Check sheet for the modelled part. Datum: model origin and axes. Units: mm. A direction names the side the tool comes from. Coordinates: 2 decimals unless noted, no trailing zeros. Loops run counter-clockwise (first coordinate to the right, second up) from the corner with the lowest first, then second, coordinate; pieces in that order, holes last. Notation, with made-up numbers: (-17, 11.25) -> (24, 11.25) arc R30 ccw to (24, 33.25) -> close; hole circle Ø10 at (34, -20.75). An arc over 180 degrees is marked (long way). Use one line per item in the form item = value.
from build123d import *

# Parameters (mm, degrees)
SKETCH2_W           = 127
SKETCH2_H           = 177.8
BOSS_EXTRUDE2_DEPTH = 5.08
SKETCH3_W           = 5.08
SKETCH3_H           = 25.4
CUT_EXTRUDE1_DEPTH  = 5.08
LPATTERN1_COUNT     = 5
LPATTERN1_PITCH     = 43.18
SKETCH4_W           = 5.08
SKETCH4_H           = 25.4
CUT_EXTRUDE2_DEPTH  = 5.08
LPATTERN2_COUNT     = 4
LPATTERN2_PITCH     = 43.18
SKETCH5_W           = 25.4
SKETCH5_H           = 5.08
CUT_EXTRUDE3_DEPTH  = 5.08
LPATTERN3_COUNT     = 3
LPATTERN3_PITCH     = 38.1
SKETCH6_W           = 25.4
SKETCH6_H           = 5.08
CUT_EXTRUDE4_DEPTH  = 5.08
LPATTERN4_COUNT     = 3
LPATTERN4_PITCH     = 38.1
SKETCH7_W           = 5.08
SKETCH7_H           = 10.16
CUT_EXTRUDE5_DEPTH  = 5.08


with BuildPart() as part:
    # Sketch2 → Boss-Extrude2 (new body)
    with BuildSketch(Plane.XY):
        with Locations((63.5, -88.9)):
            Rectangle(SKETCH2_W, SKETCH2_H)
    extrude(amount=BOSS_EXTRUDE2_DEPTH)

    # Sketch3 → Cut-Extrude1 (cut)
    with BuildSketch(Plane(origin=(0, 0, 0), x_dir=(-1, 0, 0), z_dir=(0, 0, -1))):
        with Locations((-124.46, -153.67)):
            Rectangle(SKETCH3_W, SKETCH3_H)
    cut_extrude1 = extrude(amount=-CUT_EXTRUDE1_DEPTH, mode=Mode.SUBTRACT)

    # LPattern1: Cut-Extrude1 ×5
    with Locations(*[(0, i * LPATTERN1_PITCH, 0) for i in range(1, LPATTERN1_COUNT)]):
        add(cut_extrude1, mode=Mode.SUBTRACT)

    # Sketch4 → Cut-Extrude2 (cut)
    with BuildSketch(Plane(origin=(0, 0, 0), x_dir=(-1, 0, 0), z_dir=(0, 0, -1))):
        with Locations((-2.54, -153.67)):
            Rectangle(SKETCH4_W, SKETCH4_H)
    cut_extrude2 = extrude(amount=-CUT_EXTRUDE2_DEPTH, mode=Mode.SUBTRACT)

    # LPattern2: Cut-Extrude2 ×4
    with Locations(*[(0, i * LPATTERN2_PITCH, 0) for i in range(1, LPATTERN2_COUNT)]):
        add(cut_extrude2, mode=Mode.SUBTRACT)

    # Sketch5 → Cut-Extrude3 (cut)
    with BuildSketch(Plane(origin=(0, 0, 0), x_dir=(-1, 0, 0), z_dir=(0, 0, -1))):
        with Locations((-101.6, -175.26)):
            Rectangle(SKETCH5_W, SKETCH5_H)
    cut_extrude3 = extrude(amount=-CUT_EXTRUDE3_DEPTH, mode=Mode.SUBTRACT)

    # LPattern3: Cut-Extrude3 ×3
    with Locations(*[(-i * LPATTERN3_PITCH, 0, 0) for i in range(1, LPATTERN3_COUNT)]):
        add(cut_extrude3, mode=Mode.SUBTRACT)

    # Sketch6 → Cut-Extrude4 (cut)
    with BuildSketch(Plane(origin=(0, 0, 0), x_dir=(-1, 0, 0), z_dir=(0, 0, -1))):
        with Locations((-25.4, -2.54)):
            Rectangle(SKETCH6_W, SKETCH6_H)
    cut_extrude4 = extrude(amount=-CUT_EXTRUDE4_DEPTH, mode=Mode.SUBTRACT)

    # LPattern4: Cut-Extrude4 ×3
    with Locations(*[(i * LPATTERN4_PITCH, 0, 0) for i in range(1, LPATTERN4_COUNT)]):
        add(cut_extrude4, mode=Mode.SUBTRACT)

    # Sketch7 → Cut-Extrude5 (cut)
    with BuildSketch(Plane.XY.offset(5.08)):
        with Locations((63.5, -22.86)):
            Rectangle(SKETCH7_W, SKETCH7_H)
        with Locations((63.5, -45.72)):
            Rectangle(SKETCH7_W, SKETCH7_H)
    extrude(amount=-CUT_EXTRUDE5_DEPTH, mode=Mode.SUBTRACT)


solid = part.part
(1) Section check A-A, the plane y = -45.5. Record the boundary of the cut face in (x, z), plus the area to 3 significant figures.
Established:
outline = (0, 0) -> (60.96, 0) -> (60.96, 5.08) -> (0, 5.08) -> close; (66.04, 0) -> (127, 0) -> (127, 5.08) -> (66.04, 5.08) -> close
area = 619 mm²
(2) Section check C-C, the plane x = 27. Record the boundary of the cut face in (y, z).
Established:
outline = (-172.72, 0) -> (-5.08, 0) -> (-5.08, 5.08) -> (-172.72, 5.08) -> close
(3) Section check B-B, the plane z = 3.4. Give the number of separate pieces and of enclosed holes in the cut face, plus the area to 3 significant figures.
Established:
separate_pieces = 1
enclosed_holes = 2
area = 20,700 mm²
(4) Tool access check on faces 5 (the flat face through (88.9, -3, 3)), 6 (the flat face through (3, -11.43, 3)), 7 (the flat face through (121.92, -111, 3)). Record the directions out of +Z, -Z, +X, -X, +Y, -Y that give a thin tool (end or side, any length) a straight path to the whole face; none if there is none.
Established:
face_5 = +Z, -Z, +Y
face_6 = +Z, -Z, -X
face_7 = +Z, -Z, +X
(5) Section check D-D, the plane y = -106.5. Record the boundary of the cut face in (x, z), plus the area to 3 significant figures.
Established:
outline = (5.08, 0) -> (121.92, 0) -> (121.92, 5.08) -> (5.08, 5.08) -> close
area = 594 mm²
(6) Mould release check, pull along Y, two halves, no side actions. Record for faces 1 (the flat face through (5.08, -67, 3)), 2 (the flat face through (64, -5.08, 3)), 3 (the flat face through (26, -172.72, 3)), 4 (the flat face through (0, -6, 3)): +Y half, -Y half, draft (parallel to the pull), parting line (faces both ways), or undercut.
Established:
face_1 = undercut
face_2 = +Y half
face_3 = -Y half
face_4 = draft
(7) Go/stop test with flat-tipped pins: P1, Ø2.5, axis at y = -148, z = 2, coming from the +X side; P2, Ø1.5, axis at x = 29.5, z = 2.5, coming from the -Y side; P3, Ø1, axis at x = 25, z = 0.5, coming from the +Y side. Record where each tip stops, or that it passes through.
Established:
P1 = 121.92
P2 = -172.72
P3 = -5.08
(8) Scan lines: line 1 along Y through (x, z) = (65, 0.75); line 2 along X through (y, z) = (-21.5, 3.1); line 3 along X through (y, z) = (-49.5, 4.4). Record each from-to range of solid material in increasing order.
Established:
line_1 = -172.72 to -50.8, -40.64 to -27.94, -17.78 to -5.08
line_2 = 5.08 to 60.96, 66.04 to 121.92
line_3 = 0 to 60.96, 66.04 to 127
